Read the model definition and answer for the solid it produces. Units are mm, in the model's axes. Face numbers are marked on the shaded views. A direction names the side the tool comes from. Coordinates: 2 decimals unless noted, no trailing zeros. Write each loop counter-clockwise with the first axis right and the second up, starting at its lowest first coordinate (ties: lowest second). Pieces come first, ordered by that corner, then holes.
Item 1: Section D-D (x = 75.5) is taken. Give the vertices of the cut face in (y, z), then the cut area to 3 significant figures.
Item 2: Straight lines are drawn through the part: probe 1 along Z at (x, y) = (-56, 6); probe 2 along Z at (x, y) = (25, 14.5); probe 3 along Z at (x, y) = (-5.5, -31). For each, find the intervals that lie inside material, in ascending order.
Item 3: A tool of negligible diameter and unlimited length cuts with its end or side. For the marked faces 1, 2 and 3, from which of +Z, -Z, +X, -X, +Y, -Y can it reach the whole face along a straight path? Write none if from no direction.
Item 4: Section A-A (x = -58) is taken. Give the vertices of the cut face in (y, z), then the cut area to 3 significant figures.
Item 5: Each of these flat-tipped pins is pushed along its axis until it touches: P1, Ø11.5, axis at x = -55.5, z = 166, coming from the +Y side; P2, Ø22.5, axis at x = -74.92, y = 0.92, coming from the +Z side; P3, Ø5, axis at y = -29.5, z = 71.5, coming from the -X side; P4, Ø7, axis at x = 68, z = 149, coming from the -Y side. Where does it stop, or does it pass through?
Item 6: Section C-C (z = 164) is taken. Give the vertices of the cut face in (x, y).
Item 7: Section B-B (x = 0) is taken. Give the vertices of the cut face in (y, z), then the cut area to 3 significant figures.
from build123d import *

# Parameters (mm, degrees)
F0_R      = 50
F1_DEPTH  = 300
F2_W      = 54.253433831
F2_H      = 14.4457370043
F2_W_2    = 52.9929734766
F2_H_2    = 14.163993299
F3_DEPTH  = 100
F4_W      = 57.0899797603
F4_H      = 13.7881338596
F5_DEPTH  = 100
F6_R      = 12.5
F7_DEPTH  = 158.7383495102
F8_R      = 12.5
F9_DEPTH  = 176.0267437825
F10_R     = 20
F11_R     = 20
F12_R     = 12.5
F13_DEPTH = 50
F14_R     = 12.5
F15_DEPTH = 50


with BuildPart() as f1:
    # F0 (on Top) → F1 (new body)
    with BuildSketch(Plane.XY):
        Circle(F0_R)
    extrude(amount=F1_DEPTH)

    # F2 (on Right) → F3 (join)
    with BuildSketch(Plane.YZ):
        with Locations((0.9253951721, 164.6268591285)):
            Rectangle(F2_W, F2_H)
        with Locations((0.9205453098, 131.056252867)):
            Rectangle(F2_W_2, F2_H_2)
    extrude(amount=-F3_DEPTH)

    # F4 (on Right) → F5 (join)
    with BuildSketch(Plane.YZ):
        with Locations((6.9804289378, 148.1567174196)):
            Rectangle(F4_W, F4_H)
    extrude(amount=F5_DEPTH)

    # F6 (on face) → F7 (cut, through all)
    with BuildSketch(Plane(origin=(0, 0, 141.2626504898), x_dir=(1, 0, 0), z_dir=(0, 0, -1))):
        with Locations((78.2878473401, -7.3254397139)):
            Circle(F6_R)
    extrude(amount=-F7_DEPTH, mode=Mode.SUBTRACT)

    # F8 (on face) → F9 (cut, through all)
    with BuildSketch(Plane(origin=(0, 0, 123.9742562175), x_dir=(1, 0, 0), z_dir=(0, 0, -1))):
        with Locations((-74.919745326, -0.9205453098)):
            Circle(F8_R)
    extrude(amount=-F9_DEPTH, mode=Mode.SUBTRACT)

    # F10
    f10_edges = [f1.edges().sort_by_distance(p)[0] for p in [
        (-50, 0, 300),
        (-50, 0, 0),
    ]]
    fillet(f10_edges, radius=F10_R)

    # F11
    f11_edges = [f1.edges().sort_by_distance(p)[0] for p in [
        (100, 35.525419, 148.156717),
        (100, -21.564561, 148.156717),
        (-100, -25.575941, 131.056253),
        (-100, 27.417032, 131.056253),
        (-100, -26.201322, 164.626859),
        (-100, 28.052112, 164.626859),
    ]]
    fillet(f11_edges, radius=F11_R)

    # F12 (on face) → F13 (join)
    with BuildSketch(Plane.XY.offset(300)):
        Circle(F12_R)
    extrude(amount=F13_DEPTH)

    # F14 (on face) → F15 (join)
    with BuildSketch(Plane(origin=(0, 0, 0), x_dir=(1, 0, 0), z_dir=(0, 0, -1))):
        Circle(F14_R)
    extrude(amount=F15_DEPTH)


solid = f1.part
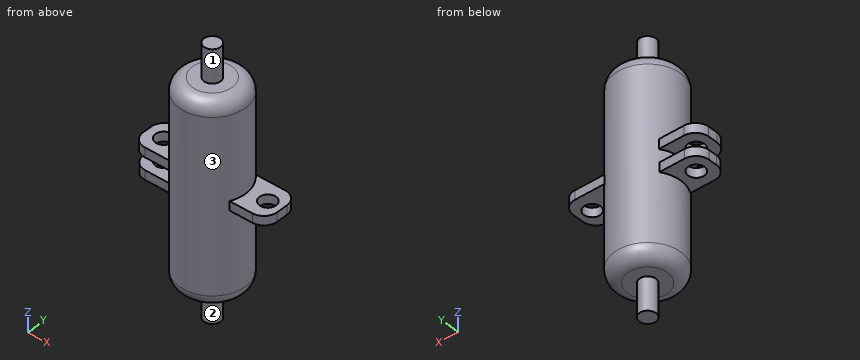
Established:
1. outline: (-21.56, 141.26) - (-4.86, 141.26) - (-4.86, 155.05) - (-21.56, 155.05) - close; (19.51, 141.26) - (35.53, 141.26) - (35.53, 155.05) - (19.51, 155.05) - close
1. area: 451 mm2
2. probe 1: z = 123.97 to 138.14, 157.4 to 171.85
2. probe 2: z = 0 to 300
2. probe 3: z = 0.06 to 299.94
3. face 1: +Z
3. face 2: -Z
3. face 3: none
4. outline: (-26.2, 157.4) - (28.05, 157.4) - (28.05, 171.85) - (-26.2, 171.85) - close; (-25.58, 123.97) - (27.42, 123.97) - (27.42, 138.14) - (-25.58, 138.14) - close
4. area: 1,530 mm2
5. P1: stops at y = 28.05
5. P2: passes through
5. P3: stops at x = -42.08
5. P4: stops at y = -21.56
6. outline: (-100, -6.2) arc R20 ccw to (-80, -26.2) - (-42.59, -26.2) arc R50 ccw (long way) to (-41.39, 28.05) - (-80, 28.05) arc R20 ccw to (-100, 8.05) - close; hole circle Ø25 at (-74.92, 0.92)
7. outline: (-50, 20) arc R20 ccw to (-30, 0) - (-12.5, 0) - (-12.5, -50) - (12.5, -50) - (12.5, 0) - (30, 0) arc R20 ccw to (50, 20) - (50, 280) arc R20 ccw to (30, 300) - (12.5, 300) - (12.5, 350) - (-12.5, 350) - (-12.5, 300) - (-30, 300) arc R20 ccw to (-50, 280) - close
7. area: 32,200 mm2
